Verification items for this drawing (mm, ordinates from the low corner). Round coordinates to 2 decimals unless told otherwise and drop trailing zeros. Write each loop counter-clockwise with the first axis right and the second up, starting at its lowest first coordinate (ties: lowest second). Pieces come first, ordered by that corner, then holes. Notation, with made-up numbers: (22.25, 17.5) -> (28.25, 17.5) arc R13 cw to (28.25, 39.5) -> close; hole circle Ø4 at (66.25, -2). An arc over 180 degrees is marked (long way). One line per item, written item: value.
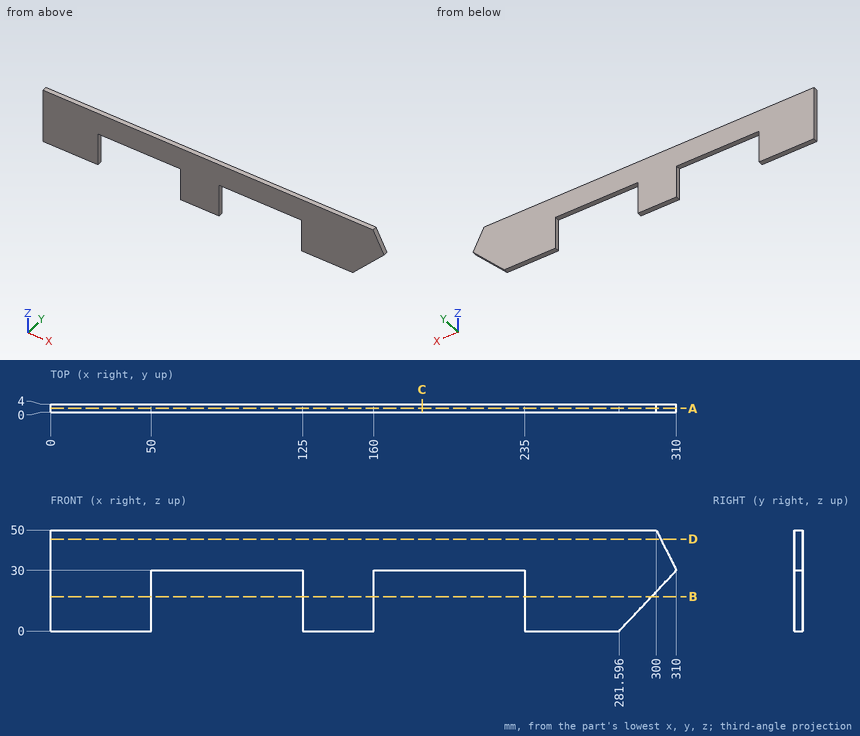
Item 1: Sectioned sample at C-C (x = 184). Enter the section's corners in (y, z).
Result set:
outline: (0, 30) -> (4, 30) -> (4, 50) -> (0, 50) -> close
Item 2: Sectioned sample at D-D (z = 45.5). Enter the section's corners in (x, y), then the cut area to 3 significant figures.
Result set:
outline: (0, 0) -> (302.25, 0) -> (302.25, 4) -> (0, 4) -> close
area: 1,210 mm^2
Item 3: Depth check by flat-ended pin: pin 1 (1.2 mm diameter, centred on y = 1.5, z = 11, fed in from +X); pin 2 (2 mm diameter, centred on x = 188, y = 2.5, fed in from -Z); pin 3 (2 mm diameter, centred on y = 2.5, z = 38.5, fed in from -X). Enter the tip coordinate at first touch or a pass-through.
Result set:
pin 1: x = 292.58
pin 2: z = 30
pin 3: x = 0
Item 4: Material ranges on line 1 along X through (y, z) = (1.2, 10.5); line 2 along X through (y, z) = (1.05, 6) (1 decimal); line 3 along Z through (x, y) = (192, 2.95), recorded low to high.
Result set:
line 1: 0 to 50, 125 to 160, 235 to 291.54
line 2: 0 to 50, 125 to 160, 235 to 287.3
line 3: 30 to 50
Item 5: Sectioned sample at B-B (z = 17). Enter the section's corners in (x, y), then the cut area to 3 significant figures.
Result set:
outline: (0, 0) -> (50, 0) -> (50, 4) -> (0, 4) -> close; (125, 0) -> (160, 0) -> (160, 4) -> (125, 4) -> close; (235, 0) -> (297.69, 0) -> (297.69, 4) -> (235, 4) -> close
area: 591 mm^2
Item 6: Sectioned sample at A-A (y = 1.85). Enter the section's corners in (x, z), then the cut area to 3 significant figures.
Result set:
outline: (0, 0) -> (50, 0) -> (50, 30) -> (125, 30) -> (125, 0) -> (160, 0) -> (160, 30) -> (235, 30) -> (235, 0) -> (281.6, 0) -> (310, 30) -> (300, 50) -> (0, 50) -> close
area: 10,500 mm^2
